Could you check a few things on this drawing? It's one solid part, dimensions in mm from its lowest x, y, z. Round coordinates to 2 decimals unless told otherwise and drop trailing zeros. Loops run counter-clockwise (first coordinate to the right, second up) from the corner with the lowest first, then second, coordinate; pieces in that order, holes last. Notation, with made-up numbers: (-1.5, -34.5) -> (16.5, -34.5) arc R12 ccw to (16.5, -30.5) -> close; hole circle Ø11 at (-8, 67.25). An arc over 180 degrees is marked (long way). Use one line per item in the form item = value. Start each with the question number.
Item 1: If I drill on L1, parallel to X at y = 2.65, z = 12.7 (3 decimals); L2, parallel to Z at x = 63.5, y = 2.1 (3 decimals); L3, parallel to X at y = 2, z = 5, over which ranges is the centre line in solid material (lowest first)? Write a range as [from, to].
Item 2: If we section it at B-B (x = 7): Write out the boundary of the cut face in (y, z).
Item 3: If we section it at A-A (y = 1.9): Write out the boundary of the cut face in (x, z) (3 decimals).
Item 4: I'm going to push a flat-ended pin straight in: pin 1 Ø5 at (x, z) = (63.5, 12.7) entering from +Y. Where does the tip first touch, or does it pass through?
Item 5: If we section it at C-C (z = 56.5): Write out the boundary of the cut face in (x, y), then the cut area to 3 significant figures.
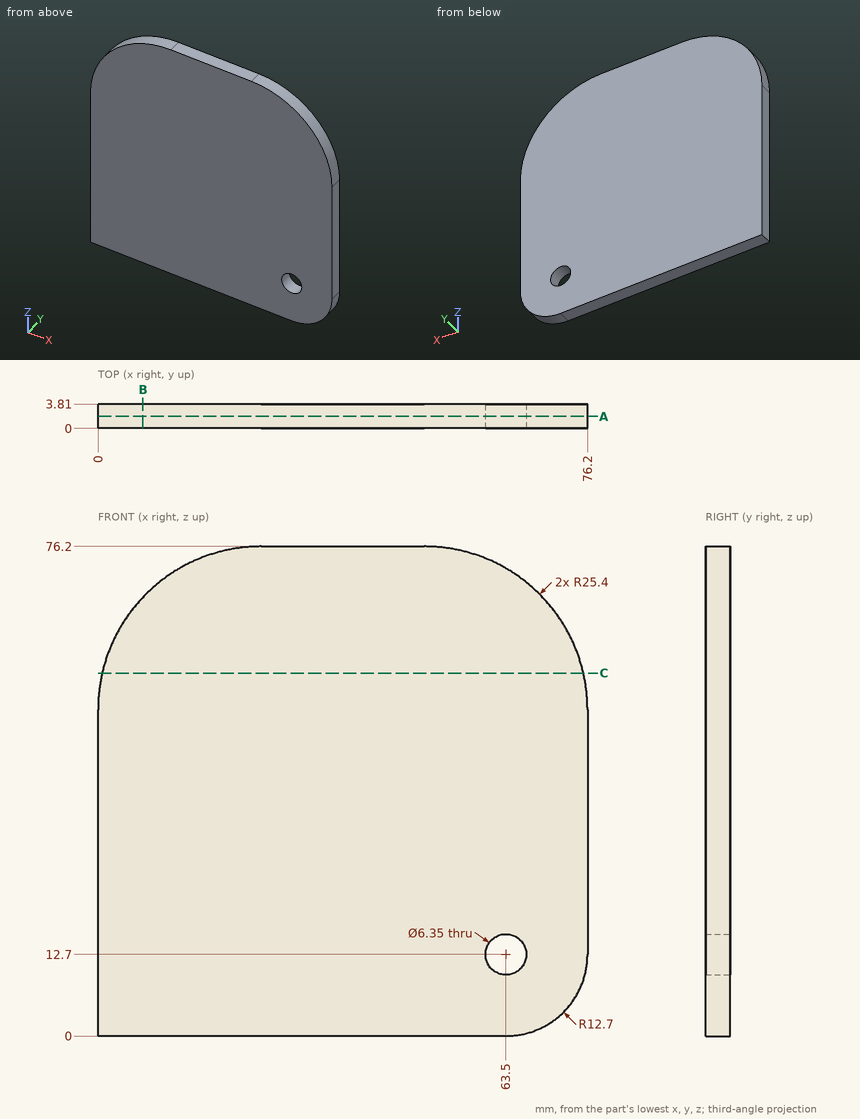
Values found:
q1.L1 = [0, 60.325], [66.675, 76.2]
q1.L2 = [0, 9.525], [15.875, 72.797]
q1.L3 = [0, 73.6]
q2.outline = (0, 0) -> (3.81, 0) -> (3.81, 68.31) -> (0, 68.31) -> close
q3.outline = (0, 0) -> (63.5, 0) arc R12.7 ccw to (76.2, 12.7) -> (76.2, 50.8) arc R25.4 ccw to (50.8, 76.2) -> (25.4, 76.2) arc R25.4 ccw to (0, 50.8) -> close; hole circle Ø6.35 at (63.5, 12.7)
q4.pin_1 = through
q5.outline = (0.65, 0) -> (75.55, 0) -> (75.55, 3.81) -> (0.65, 3.81) -> close
q5.area = 285 mm2
